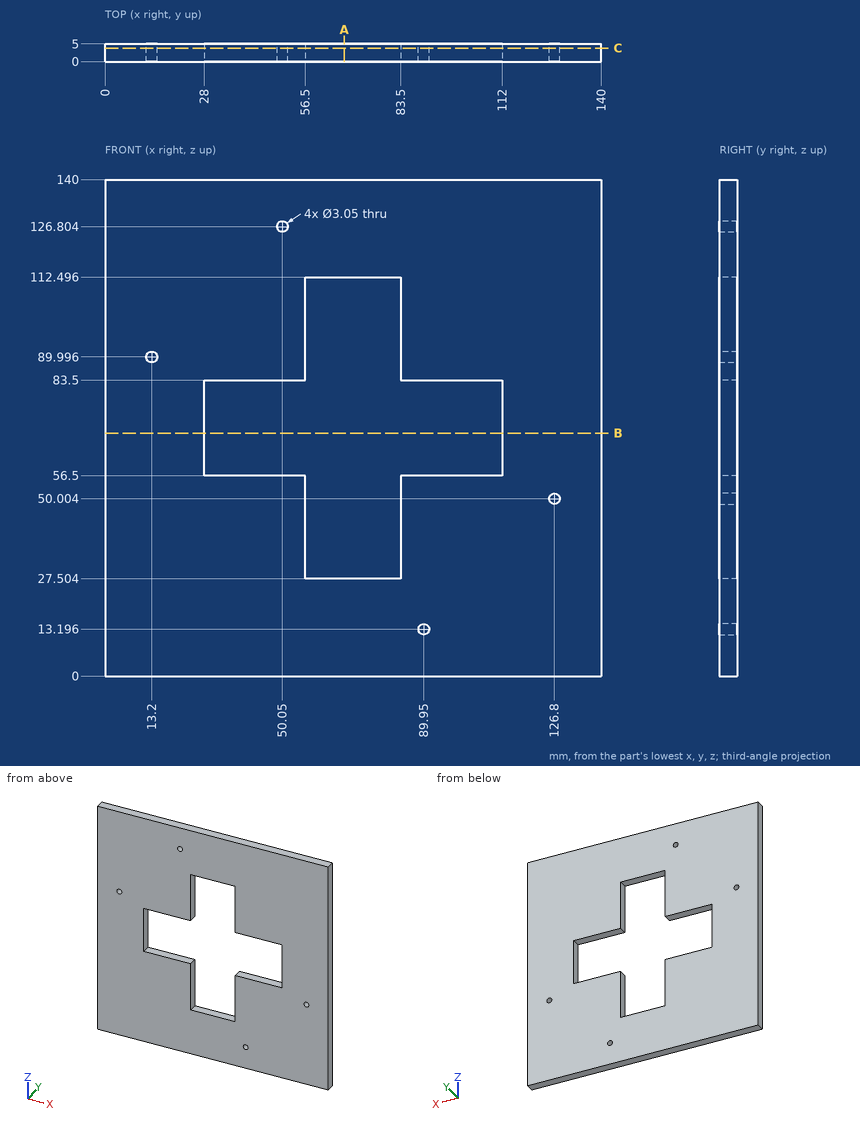
Answer from the drawing. Dimensions are ordinates in mm from the lowest x, y and z of the part. Give positions to 0.01 mm unless a question says otherwise; leave off trailing zeros. Order: outer loops, then holes, each group sorted by start corner. A loop starts at its lowest first (then second) coordinate and runs counter-clockwise, first axis right, second up.
Item 1: The part is cut by section A-A, the plane x = 67.5. Give the vertices of the cut face in (y, z) (1 decimal), and give its area (3 significant figures).
From the geometry:
outline: (0, 0) - (5, 0) - (5, 27.5) - (0, 27.5) - close; (0, 112.5) - (5, 112.5) - (5, 140) - (0, 140) - close
area: 275 mm2
Item 2: The part is cut by section B-B, the plane z = 68.5. Give the vertices of the cut face in (x, y), and give its area (3 significant figures).
From the geometry:
outline: (0, 0) - (28, 0) - (28, 5) - (0, 5) - close; (112, 0) - (140, 0) - (140, 5) - (112, 5) - close
area: 280 mm2
Item 3: Find the intervals of material crossed by probe 1 along Z at (x, y) = (89.95, 3.9); probe 2 along X at (y, z) = (1.8, 95); probe 3 along X at (y, z) = (1.2, 57), in increasing order.
From the geometry:
probe 1: z = 0 to 11.67, 14.72 to 56.5, 83.5 to 140
probe 2: x = 0 to 56.5, 83.5 to 140
probe 3: x = 0 to 28, 112 to 140
Item 4: The part is cut by section C-C, the plane y = 3.8. Count the separate pieces of the cut face and the enclosed holes in it, and give its area (3 significant figures).
From the geometry:
separate pieces: 1
enclosed holes: 5
area: 15,700 mm2
